```python
from build123d import *

# Parameters (mm, degrees)
RESSALTO_EXTRUS_O1_DEPTH   = 70
RESSALTO_EXTRUS_O4_START   = -70
RESSALTO_EXTRUS_O4_DEPTH   = 70
CASCA1_START               = 4
CASCA1_DEPTH               = 66
ESBO_O17_W                 = 10
ESBO_O17_H                 = 28
CORTE_EXTRUS_O2_DEPTH      = 10
CORTE_EXTRUS_O6_DEPTH      = 4
CORTE_EXTRUS_O6_DEPTH_BACK = 5
ESBO_O23_OUTSIDE_W         = 319.722
ESBO_O23_OUTSIDE_H         = 287.109
ESBO_O27_W                 = 5
ESBO_O27_H                 = 20
RESSALTO_EXTRUS_O5_DEPTH   = 20
FILETE2_R                  = 5
CORTE_EXTRUS_O7_DEPTH      = 104
CORTE_EXTRUS_O7_DEPTH_BACK = 5
ESBO_O28_W                 = 7.367994206
ESBO_O28_H                 = 11.845430552
ESBO_O32_R                 = 3.6
CORTE_EXTRUS_O8_DEPTH      = 187
ESBO_O32_3_R               = 9
ESBO_O32_3_R_2             = 3.6
RESSALTO_EXTRUS_O6_DEPTH   = 35
ESBO_O32_4_R               = 3.6
RESSALTO_EXTRUS_O7_DEPTH   = 6
FILETE3_R                  = 10
ESBO_O24_W                 = 73
ESBO_O24_H                 = 39
ESBO_O24_W_2               = 70
ESBO_O24_H_2               = 36
RESSALTO_EXTRUS_O8_DEPTH   = 20


# Read off the part's stored shape, not the designer's step: Casca1
with BuildPart() as part:
    # Esboço1 → Ressalto-extrusão1 (new body)
    with BuildSketch(Plane(origin=(0, 0, 0), x_dir=(1, 0, 0), z_dir=(0, 1, 0))):
        with BuildLine():
            ThreePointArc((125, 0), (-30.965140685, 121.103922572), (-109.658560997, -60))
            Line((-109.658560997, -60), (109.658560997, -60))
            ThreePointArc((109.658560997, -60), (121.103922572, -30.965140685), (125, 0))
        make_face()
    extrude(amount=RESSALTO_EXTRUS_O1_DEPTH)

    # Esboço5 → Ressalto-extrusão4 (add)
    with BuildSketch(Plane(origin=(0, 70, 0), x_dir=(1, 0, 0), z_dir=(0, 1, 0)).offset(RESSALTO_EXTRUS_O4_START)):
        with BuildLine():
            Line((-84.200220254, -92.386811338), (-78.700220254, -92.386811338))
            ThreePointArc((-78.700220254, -92.386811338), (-93.51006265, -77.362237302), (-105.49430116, -60))
            Line((-105.49430116, -60), (-109.658560997, -60))
            ThreePointArc((-109.658560997, -60), (-98.272748787, -77.249380877), (-84.200220254, -92.386811338))
        make_face()
        with BuildLine():
            Line((78.700220254, -92.386811338), (84.200220254, -92.386811338))
            ThreePointArc((84.200220254, -92.386811338), (98.272748787, -77.249380877), (109.658560997, -60))
            Line((109.658560997, -60), (105.49430116, -60))
            ThreePointArc((105.49430116, -60), (93.51006265, -77.362237302), (78.700220254, -92.386811338))
        make_face()
    extrude(amount=RESSALTO_EXTRUS_O4_DEPTH)

    # Casca1 outline → Casca1 (cut)
    with BuildSketch(Plane(origin=(0, 0, 0), x_dir=(1, 0, 0), z_dir=(0, 1, 0)).offset(CASCA1_START)):
        with BuildLine():
            Line((-107.261363034, -56), (107.261363034, -56))
            ThreePointArc((107.261363034, -56), (0, 121), (-107.261363034, -56))
        make_face()
    extrude(amount=CASCA1_DEPTH, mode=Mode.SUBTRACT)

    # Esboço17 → Corte-extrusão2 (cut)
    with BuildSketch(Plane(origin=(0, 4, 0), x_dir=(1, 0, 0), z_dir=(0, 1, 0))):
        with Locations((-105, 0)):
            Rectangle(ESBO_O17_W, ESBO_O17_H)
        with Locations((105, 0)):
            Rectangle(ESBO_O17_W, ESBO_O17_H)
    extrude(amount=-CORTE_EXTRUS_O2_DEPTH, mode=Mode.SUBTRACT)

    # Esboço23 outside → Corte-extrusão6 (cut, two sides: drawn at the far end of the back side and taken through both)
    with BuildSketch(Plane(origin=(0, 70, 0), x_dir=(1, 0, 0), z_dir=(0, 1, 0)).offset(-CORTE_EXTRUS_O6_DEPTH_BACK)):
        with Locations((0, 16.3065)):
            Rectangle(ESBO_O23_OUTSIDE_W, ESBO_O23_OUTSIDE_H)
        with BuildLine():
            Line((-108.466584716, -58), (108.466584716, -58))
            ThreePointArc((108.466584716, -58), (0, 123), (-108.466584716, -58))
        make_face(mode=Mode.SUBTRACT)
    extrude(amount=CORTE_EXTRUS_O6_DEPTH + CORTE_EXTRUS_O6_DEPTH_BACK, mode=Mode.SUBTRACT)

    # Esboço27 → Ressalto-extrusão5 (add)
    with BuildSketch(Plane.XY.offset(60)):
        with Locations((-52, 32.5)):
            Rectangle(ESBO_O27_W, ESBO_O27_H)
        with Locations((52, 32.5)):
            Rectangle(ESBO_O27_W, ESBO_O27_H)
        with Locations((0, 32.5)):
            Rectangle(ESBO_O27_W, ESBO_O27_H)
    extrude(amount=RESSALTO_EXTRUS_O5_DEPTH)

    # Filete2
    filete2_edges = [part.edges().sort_by_distance(p)[0] for p in [
        (-54.5, 32.5, 60),
        (-52, 22.5, 60),
        (-49.5, 32.5, 60),
        (-52, 42.5, 60),
        (49.5, 32.5, 60),
        (52, 22.5, 60),
        (54.5, 32.5, 60),
        (52, 42.5, 60),
        (-2.5, 32.5, 60),
        (0, 22.5, 60),
        (2.5, 32.5, 60),
        (0, 42.5, 60),
    ]]
    fillet(filete2_edges, radius=FILETE2_R)

    # Esboço28 → Corte-extrusão7 (cut, two sides: drawn at the far end of the back side and taken through both)
    with BuildSketch(Plane(origin=(-49.5, 0, 0), x_dir=(0, 0, -1), z_dir=(1, 0, 0)).offset(-CORTE_EXTRUS_O7_DEPTH_BACK)):
        with Locations((-72.5, 32.5)):
            Rectangle(ESBO_O28_W, ESBO_O28_H)
    extrude(amount=CORTE_EXTRUS_O7_DEPTH + CORTE_EXTRUS_O7_DEPTH_BACK, mode=Mode.SUBTRACT)

    # Esboço32 → Corte-extrusão8 (cut)
    with BuildSketch(Plane(origin=(0, 0, 56), x_dir=(-1, 0, 0), z_dir=(0, 0, -1))):
        with Locations(Location((0, 31.932833776, 0), (0, 0, 180))):
            Circle(ESBO_O32_R)
    extrude(amount=CORTE_EXTRUS_O8_DEPTH, mode=Mode.SUBTRACT)

    # Esboço32<3> → Ressalto-extrusão6 (add)
    with BuildSketch(Plane(origin=(0, 0, 56), x_dir=(-1, 0, 0), z_dir=(0, 0, -1))):
        with Locations((0, 31.932833776)):
            Circle(ESBO_O32_3_R)
        with Locations(Location((0, 31.932833776, 0), (0, 0, 180))):
            Circle(ESBO_O32_3_R_2, mode=Mode.SUBTRACT)
    extrude(amount=RESSALTO_EXTRUS_O6_DEPTH)

    # Esboço32<4> → Ressalto-extrusão7 (add)
    with BuildSketch(Plane(origin=(0, 0, 56), x_dir=(-1, 0, 0), z_dir=(0, 0, -1))):
        with Locations(Location((0, 31.932833776, 0), (0, 0, 180))):
            Circle(ESBO_O32_4_R)
    extrude(amount=RESSALTO_EXTRUS_O7_DEPTH)

    # Filete3
    filete3_edges = [part.edges().sort_by_distance(p)[0] for p in [
        (9, 31.932833776, 56),
    ]]
    fillet(filete3_edges, radius=FILETE3_R)

    # Esboço24 → Ressalto-extrusão8 (add)
    with BuildSketch(Plane(origin=(0, 4, 0), x_dir=(1, 0, 0), z_dir=(0, 1, 0))):
        with Locations((0, 91.008746076)):
            Rectangle(ESBO_O24_W, ESBO_O24_H)
        with Locations((0, 91.008746076)):
            Rectangle(ESBO_O24_W_2, ESBO_O24_H_2, mode=Mode.SUBTRACT)
    extrude(amount=RESSALTO_EXTRUS_O8_DEPTH)


solid = part.part
```
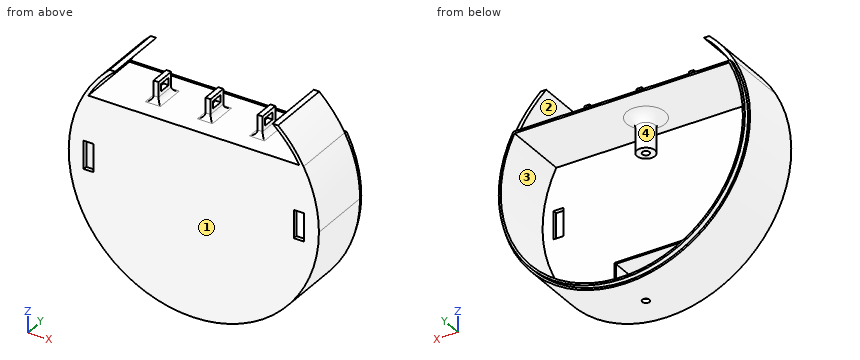
Source: CAD feature listing. Evaluate the final solid. Frame: model axes, mm. Face numbers are marked on the shaded views. A direction names the side the tool comes from. Give positions to 0.01 mm unless a question says otherwise; leave off trailing zeros. Loops run counter-clockwise (first coordinate to the right, second up) from the corner with the lowest first, then second, coordinate; pieces in that order, holes last. Notation, with made-up numbers: (-3, 14.5) -> (56, 14.5) arc R8 cw to (56, 25.5) -> close; hole circle Ø9 at (69, 2). An arc over 180 degrees is marked (long way). Use a Markdown table: item, result. Add a question column.
(1) Section query D-D (z = -7.5). Output: boundary loops of the cut face in (x, y).
(2) Section query C-C (x = 26). Output: boundary loops of the cut face in (y, z), then the cut area to 3 significant figures.
(3) Section query B-B (y = 58). Output: boundary loops of the cut face in (x, z), then the cut area to 3 significant figures.
(4) Section query A-A (z = 36.5). Output: boundary loops of the cut face in (x, y), then the cut area to 3 significant figures.
(5) First-contact query: pin 1 Ø2 at (x, y) = (-105.5, 1.5) entering from +Z; pin 2 Ø1.2 at (x, y) = (-103, 2.5) entering from -Z; pin 3 Ø1.5 at (x, z) = (53, 74) entering from +Y. Flat tips, straight axial feed; report the tip coordinate or a pass-through.
(6) Ray query, line 1 (Y direction, x = 0, z = 36); line 2 (Z direction, x = -33.5, y = 23); line 3 (X direction, y = 9, z = -105.5). Return the intervals inside material, ascending.
(7) Access query for the marked faces 3 and 4. Directions: +Z, -Z, +X, -X, +Y, -Y. A direction counts if a zero-diameter tool reaches every point of the face in a straight line with its end or side. Return the directions, or none.
(8) Pull-direction query (Z, two-part tool) for the marked faces 1 and 2; classes: +Z half, -Z half, draft (parallel to the pull), parting line (faces both ways), or undercut.
Checked values:
| question | item | result |
|---|---|---|
| 1 | outline | (-124.77, 0) -> (-110, 0) -> (-110, 4) -> (-120.77, 4) -> (-120.77, 70) -> (-122.77, 70) -> (-122.77, 65) -> (-124.77, 65) -> close; (-100, 0) -> (100, 0) -> (100, 4) -> (-100, 4) -> close; (110, 0) -> (124.77, 0) -> (124.77, 65) -> (122.77, 65) -> (122.77, 70) -> (120.77, 70) -> (120.77, 4) -> (110, 4) -> close |
| 2 | outline | (0, -122.27) -> (65, -122.27) -> (65, -120.22) -> (70, -120.22) -> (70, -118.17) -> (4, -118.17) -> (4, -110.51) -> (24, -110.51) -> (24, -109.01) -> (4, -109.01) -> (4, -73.01) -> (24, -73.01) -> (24, -71.51) -> (4, -71.51) -> (4, 56) -> (70, 56) -> (70, 58) -> (65, 58) -> (65, 60) -> (0, 60) -> close |
| 2 | area | 1,300 mm^2 |
| 3 | outline | (-105.49, 60) arc R121.36 cw to (-78.7, 92.39) -> (-84.2, 92.39) arc R125 ccw (long way) to (84.2, 92.39) -> (78.7, 92.39) arc R121.36 cw to (105.49, 60) -> close; hole (-107.26, 56) arc R121 ccw (long way) to (107.26, 56) -> close |
| 3 | area | 3,200 mm^2 |
| 4 | outline | (-119.55, 0) -> (119.55, 0) -> (119.55, 65) -> (117.46, 65) -> (117.46, 70) -> (115.36, 70) -> (115.36, 4) -> (-115.36, 4) -> (-115.36, 70) -> (-117.46, 70) -> (-117.46, 65) -> (-119.55, 65) -> close; circle Ø18 at (0, 31.93); hole circle Ø7.2 at (0, 31.93) |
| 4 | area | 1,700 mm^2 |
| 5 | pin 1 | z = 68.59 |
| 5 | pin 2 | z = -71.69 |
| 5 | pin 3 | y = 42.5 |
| 6 | line 1 | 0 to 4, 22.93 to 28.33, 35.53 to 40.93 |
| 6 | line 2 | -120.43 to -116.27, -110.51 to -109.01, -73.01 to -71.51, 56 to 60 |
| 6 | line 3 | -67.04 to -59.25, -36.5 to -35, 35 to 36.5, 59.25 to 67.04 |
| 7 | face 3 | +Y |
| 7 | face 4 | none |
| 8 | face 1 | draft |
| 8 | face 2 | undercut |
